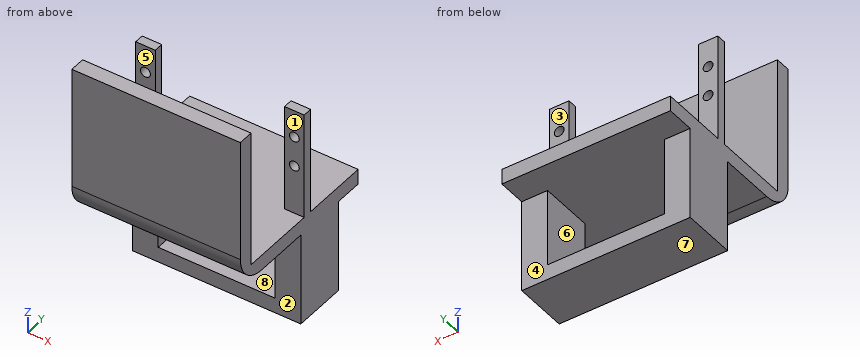
from build123d import *

# Parameters (mm, degrees)
SKETCH1_W           = 55
SKETCH1_H           = 55
BOSS_EXTRUDE1_DEPTH = 50
SKETCH2_W           = 55
SKETCH2_H           = 50
CUT_EXTRUDE1_DEPTH  = 45
FILLET2_R           = 10
SKETCH3_W           = 6.4
SKETCH3_H           = 3
BOSS_EXTRUDE2_DEPTH = 35
SKETCH4_R           = 1.6
CUT_EXTRUDE2_DEPTH  = 10
SKETCH5_W           = 8.45
SKETCH5_H           = 17.487110786
BOSS_EXTRUDE3_DEPTH = 25.4
SKETCH6_W           = 55
SKETCH6_H           = 17.487110786
BOSS_EXTRUDE4_DEPTH = 5


with BuildPart() as part:
    # Sketch1 → Boss-Extrude1 (new body)
    with BuildSketch(Plane.XY):
        with Locations((7.085987261, 0.398089172)):
            Rectangle(SKETCH1_W, SKETCH1_H)
    extrude(amount=BOSS_EXTRUDE1_DEPTH)

    # Sketch2 → Cut-Extrude1 (cut)
    with BuildSketch(Plane.XY.offset(50)):
        with Locations((7.085987261, 2.898089172)):
            Rectangle(SKETCH2_W, SKETCH2_H)
    extrude(amount=-CUT_EXTRUDE1_DEPTH, mode=Mode.SUBTRACT)

    # Fillet2
    fillet2_edges = [part.edges().sort_by_distance(p)[0] for p in [
        (7.085987261, -27.101910828, 0),
    ]]
    fillet(fillet2_edges, radius=FILLET2_R)

    # Sketch3 → Boss-Extrude2 (add)
    with BuildSketch(Plane.XY.offset(5)):
        with Locations((-17.214012739, 4.198089172)):
            Rectangle(SKETCH3_W, SKETCH3_H)
        with Locations((31.385987261, 4.198089172)):
            Rectangle(SKETCH3_W, SKETCH3_H)
    extrude(amount=BOSS_EXTRUDE2_DEPTH)

    # Sketch4 → Cut-Extrude2 (cut)
    with BuildSketch(Plane(origin=(0, 5.698089172, 0), x_dir=(1, 0, 0), z_dir=(0, 1, 0))):
        with Locations(Location((-17.214012739, -21.11, 0), (0, 0, 180))):
            Circle(SKETCH4_R)
        with Locations(Location((-17.214012739, -31.01, 0), (0, 0, 180))):
            Circle(SKETCH4_R)
        with Locations(Location((31.385987261, -31.01, 0), (0, 0, 180))):
            Circle(SKETCH4_R)
        with Locations(Location((31.385987261, -21.11, 0), (0, 0, 180))):
            Circle(SKETCH4_R)
    extrude(amount=-CUT_EXTRUDE2_DEPTH, mode=Mode.SUBTRACT)

    # Sketch5 → Boss-Extrude3 (add)
    with BuildSketch(Plane(origin=(0, 0, 0), x_dir=(-1, 0, 0), z_dir=(0, 0, -1))):
        with Locations((-30.360987261, 9.878461031)):
            Rectangle(SKETCH5_W, SKETCH5_H)
        with Locations((16.189012739, 9.878461031)):
            Rectangle(SKETCH5_W, SKETCH5_H)
    extrude(amount=BOSS_EXTRUDE3_DEPTH)

    # Sketch6 → Boss-Extrude4 (add)
    with BuildSketch(Plane(origin=(0, 0, -25.4), x_dir=(-1, 0, 0), z_dir=(0, 0, -1))):
        with Locations((-7.085987261, 9.878461031)):
            Rectangle(SKETCH6_W, SKETCH6_H)
    extrude(amount=BOSS_EXTRUDE4_DEPTH)


solid = part.part
Model file for the job. Use its own axes, mm. Face numbers are marked on the shaded views. A direction names the side the tool comes from. Give positions to 0.01 mm unless a question says otherwise; leave off trailing zeros. Loops run counter-clockwise (first coordinate to the right, second up) from the corner with the lowest first, then second, coordinate; pieces in that order, holes last.
1) Saw through at C-C (x = 7). Write the cut outline in (y, z).
2) Saw through at D-D (y = 4). Write the cut outline in (x, z), plus the area to 3 significant figures.
3) Saw through at B-B (z = -12.5). Write the cut outline in (x, y), plus the area to 3 significant figures.
4) Tool access for the marked faces 1, 2, 3 and 4: list every direction of +Z, -Z, +X, -X, +Y, -Y with a clear straight run to the whole face (end or side of a thin tool).
5) Saw through at A-A (y = 16.5). Write the cut outline in (x, z).
6) Pull direction Z, two halves, no side cores. Call the marked faces 5, 6, 7 and 8: +Z half, -Z half, draft (parallel to the pull), parting line (faces both ways), or undercut.
7) Wall check: line 1 (Z direction, x = 24, y = 8.5); line 2 (X direction, y = 14, z = -22.5); line 3 (Z direction, x = 5.5, y = -11). Give the ranges that are in metal, low to high.
8) Flat gauge pins, fed straight in: pin 1 Ø1.5 at (x, y) = (32, 4.5) entering from +Z; pin 2 Ø5 at (x, y) = (-2, 12) entering from +Z; pin 3 Ø1 at (x, y) = (-8, -8.5) entering from -Z. Where does each tip first touch, or does it go through?
Answer block:
1. outline: (-27.1, 10) arc R10 ccw to (-17.1, 0) - (27.9, 0) - (27.9, 5) - (-22.1, 5) - (-22.1, 50) - (-27.1, 50) - close; (1.13, -30.4) - (18.62, -30.4) - (18.62, -25.4) - (1.13, -25.4) - close
2. outline: (-20.41, -30.4) - (34.59, -30.4) - (34.59, 40) - (28.19, 40) - (28.19, 5) - (-14.01, 5) - (-14.01, 40) - (-20.41, 40) - close; hole circle Ø3.2 at (-17.21, 21.11); hole circle Ø3.2 at (-17.21, 31.01); hole (-11.96, -25.4) - (26.14, -25.4) - (26.14, 0) - (-11.96, 0) - close; hole circle Ø3.2 at (31.39, 21.11); hole circle Ø3.2 at (31.39, 31.01)
2. area: 1,400 mm2
3. outline: (-20.41, 1.13) - (-11.96, 1.13) - (-11.96, 18.62) - (-20.41, 18.62) - close; (26.14, 1.13) - (34.59, 1.13) - (34.59, 18.62) - (26.14, 18.62) - close
3. area: 296 mm2
4. face 1: +Z, +X, -X
4. face 2: -Z, +X, -X, -Y
4. face 3: +Z, +X, -X, +Y
4. face 4: -Z, +X, -X, +Y
5. outline: (-20.41, -30.4) - (34.59, -30.4) - (34.59, 5) - (-20.41, 5) - close; hole (-11.96, -25.4) - (26.14, -25.4) - (26.14, 0) - (-11.96, 0) - close
6. face 5: draft
6. face 6: undercut
6. face 7: -Z half
6. face 8: undercut
7. line 1: z = -30.4 to -25.4, 0 to 5
7. line 2: x = -20.41 to -11.96, 26.14 to 34.59
7. line 3: z = 0 to 5
8. pin 1: stops at z = 40
8. pin 2: stops at z = 5
8. pin 3: stops at z = 0
